```python
from build123d import *

# Parameters (mm, degrees)
BOSS_EXTRUDE1_DEPTH = 38


with BuildPart() as part:
    # Sketch1 → Boss-Extrude1 (new body)
    with BuildSketch(Plane.XY):
        with BuildLine():
            Line((66.52, 14.5), (15.54, 14.5))
            ThreePointArc((15.54, 14.5), (0.223169493, 12.66316181), (-14.225037528, 7.256815055))
            ThreePointArc((-14.225037528, 7.256815055), (-17.376400179, 0.546177113), (-11.711514098, -4.236375954))
            Line((-11.711514098, -4.236375954), (-6.590403043, -4.236765961))
            Line((-6.590403043, -4.236765961), (-6.590326886, -3.236765964))
            Line((-6.590326886, -3.236765964), (-11.687025279, -3.236377816))
            ThreePointArc((-11.687025279, -3.236377816), (-16.401861513, 0.77072863), (-13.765555848, 6.368627808))
            ThreePointArc((-13.765555848, 6.368627808), (0.459614785, 11.691517006), (15.54, 13.5))
            Line((15.54, 13.5), (66.52, 13.5))
            ThreePointArc((66.52, 13.5), (76.617843982, 8.130760845), (77.812974461, -3.243193847))
            Line((77.812974461, -3.243193847), (72.705055873, -3.242804844))
            Line((72.705055873, -3.242804844), (72.704979716, -4.242804841))
            Line((72.704979716, -4.242804841), (78.468410832, -4.243243765))
            ThreePointArc((78.468410832, -4.243243765), (77.633884428, 8.404811863), (66.52, 14.5))
        make_face()
    extrude(amount=BOSS_EXTRUDE1_DEPTH)


solid = part.part
```
For this review, take the finished solid that the model builds, in its own axes (mm). A direction names the side the tool comes from. Give positions to 0.01 mm unless a question says otherwise; leave off trailing zeros. Write each loop counter-clockwise with the first axis right and the second up, starting at its lowest first coordinate (ties: lowest second). Pieces come first, ordered by that corner, then holes. Notation, with made-up numbers: M 86,37.25 L 101,37.25 A21 cw 101,50.25 Z; hole C -32,38.25 d6. An arc over 180 degrees is marked long. Answer as a JSON object with one key per item and string values. Group by question number.
Item 1: Draft analysis for pull direction X (two halves, no side actions). For faces 4 (the cylindrical face through (-17.4, 0.66, 18.73)), 5 (the flat face through (31, 14, 38)), 6 (the cylindrical face through (76.5, 8.3, 18.7)), state which applies: +X half, -X half, draft (parallel to the pull), parting line (faces both ways), or undercut.
Item 2: For probe 1 along Y at (x, z) = (15, 34); probe 2 along Y at (x, z) = (73, 7); probe 3 along X at (y, z) = (0.5, 30), list the stretches that pass through material, from the lowest coordinate up. Write a range as [from, to].
Item 3: Tool access review of faces 1 (the cylindrical face through (0.434, 12.714, 18.734)), 2 (the cylindrical face through (-16.38, 0.68, 18.73)), 3 (the flat face through (41, 13.5, 19)): name each direction out of +Z, -Z, +X, -X, +Y, -Y from which nothing blocks a thin tool from reaching the whole face with its end or side.
Item 4: Consider section B-B on z = 28. Write out the cut boundary in (x, y).
Item 5: Consider section A-A on y = -0.75. Write out the cut boundary in (x, z).
Item 6: For pin 1 Ø2 at (y, z) = (9, 9.5) entering from +X; pin 2 Ø3 at (y, z) = (0, 33) entering from -X; pin 3 Ø2 at (y, z) = (3, 12.5) entering from +X, all flat-tipped, find the tip position at first contact; note any pin that passes through.
Item 7: Consider section D-D on x = 17. Write out the cut boundary in (y, z).
Item 8: Consider section C-C on y = 3.5. Write out the cut boundary in (x, z), plus the area to 3 significant figures.
Check result:
{
 "1": {"face 4": "-X half", "face 5": "draft", "face 6": "undercut"},
 "2": {"probe 1": "y = [13.5, 14.5]", "probe 2": "y = [-4.24, -3.24], [11.63, 12.8]", "probe 3": "x = [-17.37, -16.34], [78.67, 79.67]"},
 "3": {"face 1": "+Z, -Z, -X, +Y", "face 2": "+Z, -Z", "face 3": "+Z, -Z, -Y"},
 "4": {"outline": "M -14.23,7.26 A6.09 ccw -11.71,-4.24 L -6.59,-4.24 L -6.59,-3.24 L -11.69,-3.24 A5.09 cw -13.77,6.37 A63.78 cw 15.54,13.5 L 66.52,13.5 A12.18 cw 77.81,-3.24 L 72.71,-3.24 L 72.7,-4.24 L 78.47,-4.24 A13.18 ccw 66.52,14.5 L 15.54,14.5 A64.78 ccw Z"},
 "5": {"outline": "M -16.94,0 L -15.8,0 L -15.8,38 L -16.94,38 Z; M 78.52,0 L 79.54,0 L 79.54,38 L 78.52,38 Z"},
 "6": {"pin 1": "stops at x = 77.88", "pin 2": "stops at x = -17.51", "pin 3": "stops at x = 79.68"},
 "7": {"outline": "M 13.5,0 L 14.5,0 L 14.5,38 L 13.5,38 Z"},
 "8": {"outline": "M -17.29,0 L -16.24,0 L -16.24,38 L -17.29,38 Z; M 78.5,0 L 79.52,0 L 79.52,38 L 78.5,38 Z", "area": "78.4 mm^2"}
}
